Answer from the drawing. Dimensions are ordinates in mm from the lowest x, y and z of the part. Coordinates: 2 decimals unless noted, no trailing zeros. Loops run counter-clockwise (first coordinate to the right, second up) from the corner with the lowest first, then second, coordinate; pieces in that order, holes last. Notation, with made-up numbers: (0, 44.5) -> (19, 44.5) arc R31 ccw to (19, 75.5) -> close; hole circle Ø2 at (-32, -1). An arc over 180 degrees is marked (long way). Use a Markdown table: item, result.
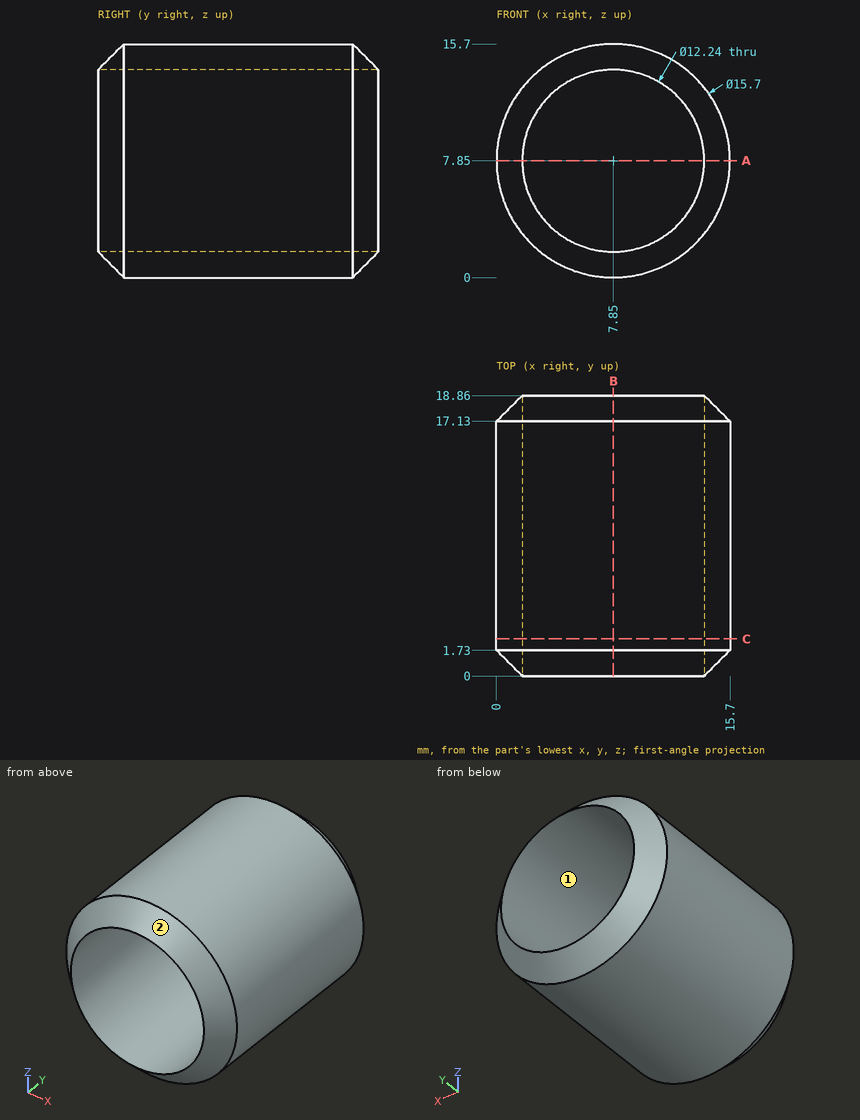
Q1. Section C-C on y = 2.5 is taken. Determine the outline of the cut face in (x, z).
Solved:
| item | result |
|---|---|
| outline | circle Ø15.7 at (7.85, 7.85); hole circle Ø12.24 at (7.85, 7.85) |
Q2. Determine the mould class of the marked faces 1 and 2 for opening direction Z: pulls with the +Z half, pulls with the -Z half, needs draft (parallel to the pull), parting line crosses it, or undercut.
Solved:
| item | result |
|---|---|
| face 1 | undercut |
| face 2 | parting line crosses it |
Q3. Consider line 1 (Z direction, x = 7.85, y = 14.5); line 2 (X direction, y = 17.75, z = 7); line 3 (Z direction, x = 3.75, y = 8.5). Determine where each line is inside the solid, lowest interval first. Write a range as [from, to].
Solved:
| item | result |
|---|---|
| line 1 | [0, 1.73], [13.97, 15.7] |
| line 2 | [0.67, 1.79], [13.91, 15.03] |
| line 3 | [1.16, 3.31], [12.39, 14.54] |
Q4. Section B-B on x = 7.85 is taken. Determine the outline of the cut face in (y, z), and give its area (3 significant figures).
Solved:
| item | result |
|---|---|
| outline | (0, 1.73) -> (1.73, 0) -> (17.13, 0) -> (18.86, 1.73) -> close; (0, 13.97) -> (18.86, 13.97) -> (17.13, 15.7) -> (1.73, 15.7) -> close |
| area | 59.3 mm² |
Q5. Given pin 1 Ø6 at (x, y) = (1.5, 9.5) entering from -Z; pin 2 Ø2 at (y, z) = (3.5, 5) entering from -X; pin 3 Ø4 at (x, z) = (8, 10.5) entering from -Y; pin 4 Ø4 at (y, z) = (13.5, 5.5) entering from +X, each flat-ended and moving along its own axis, determine where each tip first touches the part or whether it passes through.
Solved:
| item | result |
|---|---|
| pin 1 | z = 0.75 |
| pin 2 | x = 0.22 |
| pin 3 | through |
| pin 4 | x = 15.69 |
Q6. Section A-A on z = 7.85 is taken. Determine the outline of the cut face in (x, y), and give its area (3 significant figures).
Solved:
| item | result |
|---|---|
| outline | (0, 1.73) -> (1.73, 0) -> (1.73, 18.86) -> (0, 17.13) -> close; (13.97, 0) -> (15.7, 1.73) -> (15.7, 17.13) -> (13.97, 18.86) -> close |
| area | 59.3 mm² |
